Check sheet for the drawn part. Datum: minimum x, y, z corner. Units: mm. A direction names the side the tool comes from. Give positions to 0.01 mm unless a question says otherwise; leave off trailing zeros. Write each loop counter-clockwise with the first axis right and the second up, starting at its lowest first coordinate (ties: lowest second). Pieces come first, ordered by that corner, then holes. Notation, with made-up numbers: (37, 9) - (77, 9) arc R8 cw to (77, 15) - close; hole circle Ø5 at (89, 8). An arc over 180 degrees is marked (long way). Use a Markdown table: item, result.
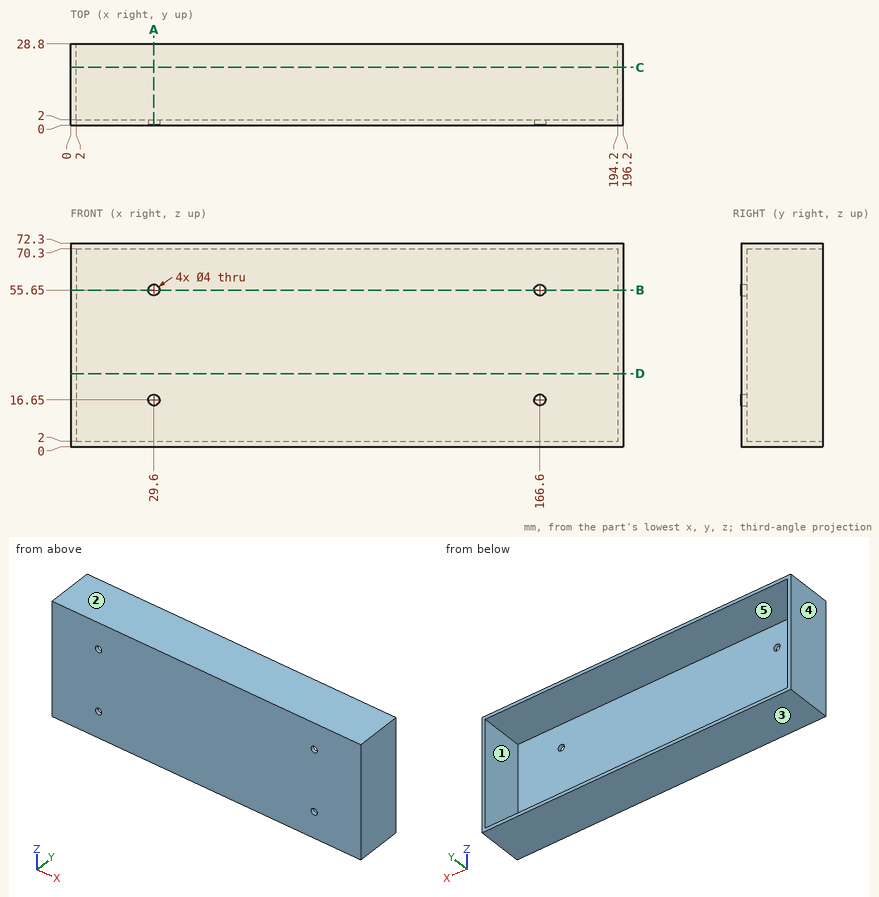
1) Section check C-C on y = 20.5. Record the boundary of the cut face in (x, z), then the cut area to 3 significant figures.
Working result:
| item | result |
|---|---|
| outline | (0, 0) - (196.2, 0) - (196.2, 72.3) - (0, 72.3) - close; hole (2, 2) - (194.2, 2) - (194.2, 70.3) - (2, 70.3) - close |
| area | 1,060 mm² |
2) Depth check by flat-ended pin: P1, Ø1.5, axis at x = 142.5, z = 62.5, coming from the +Y side; P2, Ø4, axis at y = 15, z = 30.5, coming from the -X side. Enter the tip coordinate at first touch or a pass-through.
Working result:
| item | result |
|---|---|
| P1 | stops at y = 2 |
| P2 | stops at x = 0 |
3) Set-up check for the marked faces 1 and 2: record each of +Z, -Z, +X, -X, +Y, -Y from which the full face is reachable in a straight line by a thin tool's end or side.
Working result:
| item | result |
|---|---|
| face 1 | +Y |
| face 2 | +Z, +X, -X, +Y, -Y |
4) Mould release check, pull along Z, two halves, no side actions. Record for the marked faces 3, 4 and 5: pulls with the +Z half, pulls with the -Z half, needs draft (parallel to the pull), parting line crosses it, or undercut.
Working result:
| item | result |
|---|---|
| face 3 | pulls with the -Z half |
| face 4 | needs draft |
| face 5 | undercut |
5) Section check A-A on x = 29.6. Record the boundary of the cut face in (y, z), then the cut area to 3 significant figures.
Working result:
| item | result |
|---|---|
| outline | (0, 0) - (28.8, 0) - (28.8, 2) - (2, 2) - (2, 14.65) - (0, 14.65) - close; (0, 18.65) - (2, 18.65) - (2, 53.65) - (0, 53.65) - close; (0, 57.65) - (2, 57.65) - (2, 70.3) - (28.8, 70.3) - (28.8, 72.3) - (0, 72.3) - close |
| area | 236 mm² |
6) Material ranges on L1, parallel to X at y = 1.55, z = 16.65; L2, parallel to X at y = 12, z = 32.5; L3, parallel to Z at x = 135, y = 21.25, recorded low to high. Write a range as from..to.
Working result:
| item | result |
|---|---|
| L1 | x = 0..27.6, 31.6..164.6, 168.6..196.2 |
| L2 | x = 0..2, 194.2..196.2 |
| L3 | z = 0..2, 70.3..72.3 |
7) Section check D-D on z = 26. Record the boundary of the cut face in (x, y).
Working result:
| item | result |
|---|---|
| outline | (0, 0) - (196.2, 0) - (196.2, 28.8) - (194.2, 28.8) - (194.2, 2) - (2, 2) - (2, 28.8) - (0, 28.8) - close |
8) Section check B-B on z = 55.65. Record the boundary of the cut face in (x, y).
Working result:
| item | result |
|---|---|
| outline | (0, 0) - (27.6, 0) - (27.6, 2) - (2, 2) - (2, 28.8) - (0, 28.8) - close; (31.6, 0) - (164.6, 0) - (164.6, 2) - (31.6, 2) - close; (168.6, 0) - (196.2, 0) - (196.2, 28.8) - (194.2, 28.8) - (194.2, 2) - (168.6, 2) - close |
